Part model, mm, in its own coordinate system. A direction names the side the tool comes from. Give positions to 0.01 mm unless a question says otherwise; leave off trailing zeros. Write each loop counter-clockwise with the first axis right and the second up, starting at its lowest first coordinate (ties: lowest second). Pieces come first, ordered by that corner, then holes.
```python
from build123d import *

# Parameters (mm, degrees)
IZIM1_R                     = 19.05
IZIM1_R_2                   = 2.55
IZIM1_R_3                   = 4
Y_KSEKLIK_EKSTR_ZYON1_DEPTH = 4.8
Y_KSEKLIK_EKSTR_ZYON2_DEPTH = 1.6
IZIM3_R                     = 4
Y_KSEKLIK_EKSTR_ZYON3_DEPTH = 19.4
KES_EKSTR_ZYON1_DEPTH       = 15
Y_KSEKLIK_EKSTR_ZYON4_DEPTH = 77.2
RADYUS1_R                   = 0.5


with BuildPart() as part:
    # Çizim1 → Yükseklik-Ekstrüzyon1 (new body)
    # profile 1 of 3: a face of its own
    with BuildSketch(Plane.XY):
        with BuildLine():
            Line((-34.313511383, 32.517298381), (14.686488617, 32.517298381))
            ThreePointArc((14.686488617, 32.517298381), (17.514915741, 31.345725506), (18.686488617, 28.517298381))
            Line((18.686488617, 28.517298381), (18.686488617, -20.482701619))
            ThreePointArc((18.686488617, -20.482701619), (17.514915741, -23.311128744), (14.686488617, -24.482701619))
            Line((14.686488617, -24.482701619), (-34.313511383, -24.482701619))
            ThreePointArc((-34.313511383, -24.482701619), (-37.141938508, -23.311128744), (-38.313511383, -20.482701619))
            Line((-38.313511383, -20.482701619), (-38.313511383, 28.517298381))
            ThreePointArc((-38.313511383, 28.517298381), (-37.141938508, 31.345725506), (-34.313511383, 32.517298381))
        make_face()
        with Locations((-9.813511383, 4.017298381)):
            Circle(IZIM1_R, mode=Mode.SUBTRACT)
        with Locations((13.756488617, 27.587298381)):
            Circle(IZIM1_R_2, mode=Mode.SUBTRACT)
        with Locations((13.756488617, -19.552701619)):
            Circle(IZIM1_R_2, mode=Mode.SUBTRACT)
        with Locations((-33.383511383, -19.552701619)):
            Circle(IZIM1_R_2, mode=Mode.SUBTRACT)
        with Locations((-33.383511383, 27.587298381)):
            Circle(IZIM1_R_2, mode=Mode.SUBTRACT)
    # profile 2 of 3: a face of its own
    with BuildSketch(Plane.XY):
        with Locations((-9.813511383, 4.017298381)):
            Circle(IZIM1_R)
        with Locations((-9.813511383, 4.017298381)):
            Circle(IZIM1_R_3, mode=Mode.SUBTRACT)
    # profile 3 of 3: a face of its own
    with BuildSketch(Plane.XY):
        with Locations((-9.813511383, 4.017298381)):
            Circle(IZIM1_R_3)
    extrude(amount=-Y_KSEKLIK_EKSTR_ZYON1_DEPTH)

    # Çizim2 → Yükseklik-Ekstrüzyon2 (add)
    with BuildSketch(Plane.XY):
        with BuildLine():
            ThreePointArc((9.186488617, 4.017298381), (3.621517459, 17.452327223), (-9.813511383, 23.017298381))
            Line((-9.813511383, 23.017298381), (-9.813511383, -14.982701619))
            ThreePointArc((-9.813511383, -14.982701619), (3.621517459, -9.417730462), (9.186488617, 4.017298381))
        make_face()
        with BuildLine():
            Line((-9.813511383, -14.982701619), (-9.813511383, 23.017298381))
            ThreePointArc((-9.813511383, 23.017298381), (-28.813511383, 4.017298381), (-9.813511383, -14.982701619))
        make_face()
    extrude(amount=Y_KSEKLIK_EKSTR_ZYON2_DEPTH)

    # Çizim3 → Yükseklik-Ekstrüzyon3 (add)
    with BuildSketch(Plane.XY.offset(1.6)):
        with Locations((-9.813511383, 4.017298381)):
            Circle(IZIM3_R)
    extrude(amount=Y_KSEKLIK_EKSTR_ZYON3_DEPTH)

    # Çizim4 → Kes-Ekstrüzyon1 (cut)
    with BuildSketch(Plane.XY.offset(21)):
        Polygon((-6.313511383, 4.017298381), (-6.313511383, 6.245974497), (-5.024546615, 6.245974497), (-5.024546615, 1.577201368), (-6.313511383, 1.577201368), align=None)
    extrude(amount=-KES_EKSTR_ZYON1_DEPTH, mode=Mode.SUBTRACT)

    # Çizim5 → Yükseklik-Ekstrüzyon4 (add)
    with BuildSketch(Plane(origin=(0, 0, -4.8), x_dir=(-1, 0, 0), z_dir=(0, 0, -1))):
        with BuildLine():
            ThreePointArc((-8.826488617, 27.587298381), (-10.270452185, 24.10126195), (-13.756488617, 22.657298381))
            Line((-13.756488617, 22.657298381), (-13.756488617, -14.622701619))
            ThreePointArc((-13.756488617, -14.622701619), (-10.270452185, -16.066665188), (-8.826488617, -19.552701619))
            Line((-8.826488617, -19.552701619), (28.453511383, -19.552701619))
            ThreePointArc((28.453511383, -19.552701619), (29.897474952, -16.066665188), (33.383511383, -14.622701619))
            Line((33.383511383, -14.622701619), (33.383511383, 22.657298381))
            ThreePointArc((33.383511383, 22.657298381), (29.897474952, 24.10126195), (28.453511383, 27.587298381))
            Line((28.453511383, 27.587298381), (-8.826488617, 27.587298381))
        make_face()
    extrude(amount=Y_KSEKLIK_EKSTR_ZYON4_DEPTH)

    # Radyus1
    radyus1_edges = [part.edges().sort_by_distance(p)[0] for p in [
        (-37.141938508, 31.345725506, -4.8),
        (-38.313511383, 4.017298381, -4.8),
        (-37.141938508, -23.311128744, -4.8),
        (-9.813511383, -24.482701619, -4.8),
        (17.514915741, -23.311128744, -4.8),
        (18.686488617, 4.017298381, -4.8),
        (17.514915741, 31.345725506, -4.8),
        (-37.141938508, 31.345725506, 0),
        (-38.313511383, 4.017298381, 0),
        (-37.141938508, -23.311128744, 0),
        (-9.813511383, -24.482701619, 0),
        (17.514915741, -23.311128744, 0),
        (18.686488617, 4.017298381, 0),
        (17.514915741, 31.345725506, 0),
        (-28.453511383, 27.587298381, -43.4),
        (-33.383511383, 22.657298381, -43.4),
        (-33.383511383, -14.622701619, -43.4),
        (-29.897474952, -16.066665188, -82),
        (-28.453511383, -19.552701619, -43.4),
        (-9.813511383, -19.552701619, -82),
        (10.270452185, -16.066665188, -82),
        (8.826488617, -19.552701619, -43.4),
        (13.756488617, -14.622701619, -43.4),
        (-9.813511383, 27.587298381, -82),
        (8.826488617, 27.587298381, -43.4),
        (10.270452185, 24.10126195, -82),
        (13.756488617, 22.657298381, -43.4),
        (13.756488617, 4.017298381, -82),
        (-13.813511383, 4.017298381, 21),
        (-9.813511383, 32.517298381, -4.8),
        (-9.813511383, 32.517298381, 0),
    ]]
    fillet(radyus1_edges, radius=RADYUS1_R - 0.0001)  # a hair under: the kernel refuses the full size


solid = part.part
```
1) 3-axis set-ups, long thin cutter, end or side, ignore diameter. For faces 5 (the face through (-30, 24, -43)), 6 (the face through (-10, -19.553, -43)), 7 (the face through (-13.81, 4.19, 10.92)), 8 (the face through (10.304, -16.033, -42.613)), 9 (the face through (-10, 29, -4.8)): which of +Z, -Z, +X, -X, +Y, -Y reach the whole face in a straight line?
Answers follow:
face 5: -Z, -X, +Y
face 6: -Z, +X, -X, -Y
face 7: +Z
face 8: -Z, +X, -Y
face 9: -Z
2) Saw through at B-B, the plane z = -74. Write the cut outline in (x, y), then the cut area to 3 significant figures.
Answers follow:
outline: (-33.38, -14.15) arc R0.5 ccw to (-32.93, -14.64) arc R4.93 cw to (-28.47, -19.1) arc R0.5 ccw to (-27.98, -19.55) - (8.35, -19.55) arc R0.5 ccw to (8.85, -19.1) arc R4.93 cw to (13.3, -14.64) arc R0.5 ccw to (13.76, -14.15) - (13.76, 22.18) arc R0.5 ccw to (13.3, 22.68) arc R4.93 cw to (8.85, 27.13) arc R0.5 ccw to (8.35, 27.59) - (-27.98, 27.59) arc R0.5 ccw to (-28.47, 27.13) arc R4.93 cw to (-32.93, 22.68) arc R0.5 ccw to (-33.38, 22.18) - close
area: 2,150 mm2
3) Saw through at D-D, the plane y = 20. Write the cut outline in (x, z), then the cut area to 3 significant figures.
Answers follow:
outline: (-38.31, -4.3) arc R0.5 ccw to (-37.81, -4.8) - (-33.38, -4.8) - (-33.38, -82) - (13.26, -82) arc R0.5 ccw to (13.76, -81.5) - (13.76, -4.8) - (18.19, -4.8) arc R0.5 ccw to (18.69, -4.3) - (18.69, -0.5) arc R0.5 ccw to (18.19, 0) - (0.46, 0) - (0.46, 1.6) - (-20.09, 1.6) - (-20.09, 0) - (-37.81, 0) arc R0.5 ccw to (-38.31, -0.5) - close
area: 3,950 mm2
4) Pin check, flat tips, straight feed: pin 1 Ø11 at (x, z) = (-13, -28) entering from +Y; pin 2 Ø3 at (x, y) = (13.76, -19.55) entering from +Z; pin 3 Ø6 at (x, z) = (-14, -36.5) entering from -Y; pin 4 Ø8 at (x, y) = (-33.38, 27.59) entering from -Z. Stop position of each tip, or through.
Answers follow:
pin 1: stops at y = 27.59
pin 2: passes through
pin 3: stops at y = -19.55
pin 4: stops at z = -4.8
5) Wall check: L1, parallel to X at y = -4, z = -51.5; L2, parallel to Z at x = -34, y = 9; L3, parallel to Z at x = -18.5, y = -1.5. Give the ranges that are in metal, low to high.
Answers follow:
L1: x = -33.38 to 13.76
L2: z = -4.8 to 0
L3: z = -82 to 1.6
6) Saw through at A-A, the plane y = 12. Write the cut outline in (x, z), then the cut area to 3 significant figures.
Answers follow:
outline: (-38.31, -4.3) arc R0.5 ccw to (-37.81, -4.8) - (-33.38, -4.8) - (-33.38, -82) - (13.26, -82) arc R0.5 ccw to (13.76, -81.5) - (13.76, -4.8) - (18.19, -4.8) arc R0.5 ccw to (18.69, -4.3) - (18.69, -0.5) arc R0.5 ccw to (18.19, 0) - (7.43, 0) - (7.43, 1.6) - (-27.06, 1.6) - (-27.06, 0) - (-37.81, 0) arc R0.5 ccw to (-38.31, -0.5) - close
area: 3,970 mm2
7) Two-plate mould, pull along X, no slides. Class faces 1 (the face through (-33.715, -17.024, -2.366)), 2 (the face through (-38.314, 4, -2)), 3 (the face through (-10, 4, 21)), 4 (the face through (13.425, 30.116, -2.366)): +X half, -X half, draft (parallel to the pull), parting line (faces both ways), or undercut.
Answers follow:
face 1: undercut
face 2: -X half
face 3: draft
face 4: undercut
8) Saw through at C-C, the plane x = -24.5. Write the cut outline in (y, z).
Answers follow:
outline: (-24.48, -4.3) arc R0.5 ccw to (-23.98, -4.8) - (-19.55, -4.8) - (-19.55, -81.5) arc R0.5 ccw to (-19.05, -82) - (27.09, -82) arc R0.5 ccw to (27.59, -81.5) - (27.59, -4.8) - (32.02, -4.8) arc R0.5 ccw to (32.52, -4.3) - (32.52, -0.5) arc R0.5 ccw to (32.02, 0) - (16.07, 0) - (16.07, 1.6) - (-8.04, 1.6) - (-8.04, 0) - (-23.98, 0) arc R0.5 ccw to (-24.48, -0.5) - close
